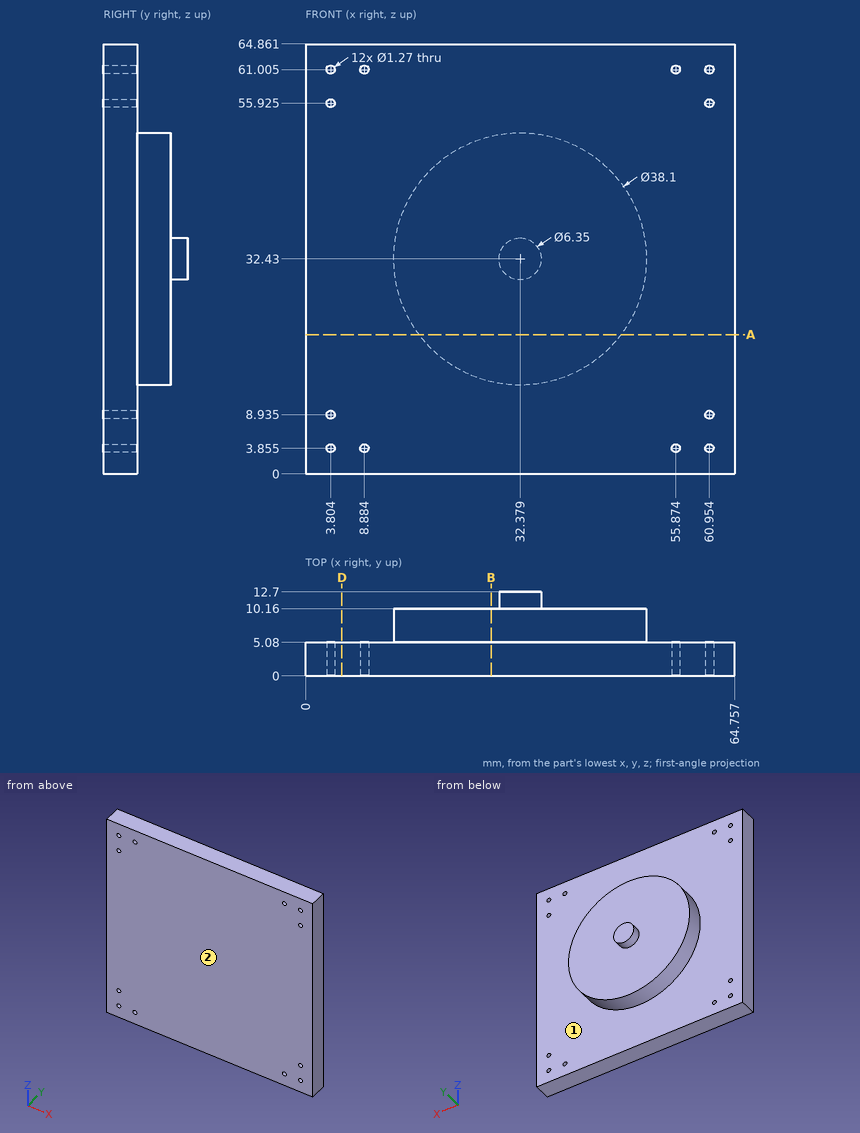
For this review, use the dimensioned drawing (mm, ordinates from the lowest corner) and the shaded views. A direction names the side the tool comes from. Round coordinates to 2 decimals unless told otherwise and drop trailing zeros. Order: outer loops, then holes, each group sorted by start corner. A loop starts at its lowest first (then second) coordinate and runs counter-clockwise, first axis right, second up. Notation, with made-up numbers: M 20.5,-35.75 L 68.5,-35.75 A22 cw 68.5,0.25 Z; hole C 27.5,62 d9. An arc over 180 degrees is marked long. Write each question's results on one line, items separated by ' | '. Start each with the question number.
1. To check wall thickness, follow L1, parallel to Z at x = 61, y = 1; L2, parallel to X at y = 8.5, z = 32; L3, parallel to Y at x = 8.5, z = 9.5. State the ranges of each line that lie inside material, in increasing order. Write a range as [from, to].
2. Clearance check with flat-ended pins moving along their axes: pin 1 Ø1.5 at (x, z) = (8.88, 3.86) entering from +Y; pin 2 Ø1.5 at (x, z) = (3.8, 55.93) entering from -Y; pin 3 Ø0.8 at (x, z) = (8.88, 61.01) entering from -Y. State where each tip first meets the part, or that it passes through.
3. Add section B-B (x = 28). State the section outline as (y, z) points, then the cut area to 3 significant figures.
4. Add section D-D (x = 5.5). State the section outline as (y, z) points.
5. Add section A-A (z = 21). State the section outline as (x, y) points.
6. Tool access review of the marked faces 1 and 2: name each direction out of +Z, -Z, +X, -X, +Y, -Y from which nothing blocks a thin tool from reaching the whole face with its end or side.
Output values:
1) L1: [0, 3.22], [4.49, 8.3], [9.57, 55.29], [56.56, 60.37], [61.64, 64.86] | L2: [13.33, 51.42] | L3: [0, 5.08]
2) pin 1: y = 5.08 | pin 2: y = 0 | pin 3: through
3) outline: M 0,0 L 5.08,0 L 5.08,13.89 L 10.16,13.89 L 10.16,50.97 L 5.08,50.97 L 5.08,64.86 L 0,64.86 Z | area: 518 mm^2
4) outline: M 0,0 L 5.08,0 L 5.08,64.86 L 0,64.86 Z
5) outline: M 0,0 L 64.76,0 L 64.76,5.08 L 47.62,5.08 L 47.62,10.16 L 17.14,10.16 L 17.14,5.08 L 0,5.08 Z
6) face 1: +Y | face 2: +Z, -Z, +X, -X, -Y
